from build123d import *

# Parameters (mm, degrees)
CROQUIS1_R              = 33
SALIENTE_EXTRUIR1_DEPTH = 10
VACIADO1_T              = -3
REDONDEO1_R             = 5
CORTAR_EXTRUIR1_REACH   = 49.728
CROQUIS2_R              = 1.25
CHAFL_N1_SIZE           = 1.6


with BuildPart() as part:
    # Croquis1 → Saliente-Extruir1 (new body)
    with BuildSketch(Plane.XY):
        Circle(CROQUIS1_R)
    extrude(amount=SALIENTE_EXTRUIR1_DEPTH)

    # Vaciado1
    vaciado1_openings = [part.faces().sort_by_distance(p)[0] for p in [
        (0, 0, 0),
    ]]
    offset(amount=VACIADO1_T, openings=vaciado1_openings, kind=Kind.INTERSECTION)

    # Redondeo1
    redondeo1_edges = [part.edges().sort_by_distance(p)[0] for p in [
        (-33, 0, 10),
        (-30, 0, 7),
    ]]
    fillet(redondeo1_edges, radius=REDONDEO1_R)

    # Croquis2 → Cortar-Extruir1 (cut, up to next)
    with BuildSketch(Plane.XY.offset(10), mode=Mode.PRIVATE) as cortar_extruir1_sk1:
        with Locations((14.041823927, -17.282568698)):
            Circle(CROQUIS2_R)
    cortar_extruir1_tool1 = extrude(cortar_extruir1_sk1.sketch, amount=-CORTAR_EXTRUIR1_REACH, mode=Mode.PRIVATE) & part.part
    # Croquis2 → Cortar-Extruir1 (cut, up to next)
    with BuildSketch(Plane.XY.offset(10), mode=Mode.PRIVATE) as cortar_extruir1_sk2:
        with Locations((19.215864901, 11.252134735)):
            Circle(CROQUIS2_R)
    cortar_extruir1_tool2 = extrude(cortar_extruir1_sk2.sketch, amount=-CORTAR_EXTRUIR1_REACH, mode=Mode.PRIVATE) & part.part
    # Croquis2 → Cortar-Extruir1 (cut, up to next)
    with BuildSketch(Plane.XY.offset(10), mode=Mode.PRIVATE) as cortar_extruir1_sk3:
        with Locations((-19.215864901, -11.252134735)):
            Circle(CROQUIS2_R)
    cortar_extruir1_tool3 = extrude(cortar_extruir1_sk3.sketch, amount=-CORTAR_EXTRUIR1_REACH, mode=Mode.PRIVATE) & part.part
    # Croquis2 → Cortar-Extruir1 (cut, up to next)
    with BuildSketch(Plane.XY.offset(10), mode=Mode.PRIVATE) as cortar_extruir1_sk4:
        with Locations((-14.041823927, 17.282568698)):
            Circle(CROQUIS2_R)
    cortar_extruir1_tool4 = extrude(cortar_extruir1_sk4.sketch, amount=-CORTAR_EXTRUIR1_REACH, mode=Mode.PRIVATE) & part.part
    add(cortar_extruir1_tool1.solids().sort_by_distance((14.041824, -17.282569, 10))[0], mode=Mode.SUBTRACT)
    add(cortar_extruir1_tool2.solids().sort_by_distance((19.215865, 11.252135, 10))[0], mode=Mode.SUBTRACT)
    add(cortar_extruir1_tool3.solids().sort_by_distance((-19.215865, -11.252135, 10))[0], mode=Mode.SUBTRACT)
    add(cortar_extruir1_tool4.solids().sort_by_distance((-14.041824, 17.282569, 10))[0], mode=Mode.SUBTRACT)

    # Chaflán1
    chafl_n1_edges = [part.edges().sort_by_distance(p)[0] for p in [
        (12.791823927, -17.282568698, 10),
        (17.965864901, 11.252134735, 10),
        (-20.465864901, -11.252134735, 10),
        (-15.291823927, 17.282568698, 10),
    ]]
    chamfer(chafl_n1_edges, length=CHAFL_N1_SIZE)


solid = part.part
Verification items for the finished model (mm, model axes). A direction names the side the tool comes from. Round coordinates to 2 decimals unless told otherwise and drop trailing zeros. Loops run counter-clockwise (first coordinate to the right, second up) from the corner with the lowest first, then second, coordinate; pieces in that order, holes last. Notation, with made-up numbers: (82, 56.25) - (132, 56.25) arc R21 ccw to (132, 66.25) - close; hole circle Ø6 at (14, -37). An arc over 180 degrees is marked (long way). Answer in a Markdown table with one row per item. Add a question column.
Q1. Section check C-C on z = 3. Enter the section's corners in (x, y), plus the area to 3 significant figures.
Q2. Tool access check on faces 5 (the face through (-29.97, 1.32, 0.99)), 6 (the face through (13.12, -16.44, 7.71)). Record the directions out of +Z, -Z, +X, -X, +Y, -Y that give a thin tool (end or side, any length) a straight path to the whole face; none if there is none.
Q3. Gauge pin test, flat ends, axial feed: pin 1 (5 mm diameter, centred on y = 23.5, z = 3, fed in from -X); pin 2 (25 mm diameter, centred on x = 0.5, y = 6.5, fed in from -Z); pin 3 (3 mm diameter, centred on x = -19.22, y = -11.25, fed in from +Z); pin 4 (1.5 mm diameter, centred on x = 14.04, y = -17.28, fed in from -Z). Record the tip position at first contact, or that the pin passes through.
Q4. Section check A-A on x = 0. Enter the section's corners in (y, z).
Q5. Release check for a two-part mould opening along Y. For faces 1 (the face through (20.37, 10.77, 7.71)), 2 (the face through (30.5, -12.6, 2.5)), 3 (the face through (0, 0, 7)), 4 (the face through (15, -27, 0)) record: pulls with the +Y half, pulls with the -Y half, needs draft (parallel to the pull), parting line crosses it, or undercut.
Q6. Material ranges on line 1 (Z direction, x = 0.5, y = 10.5); line 2 (Y direction, x = -15, z = 3); line 3 (Y direction, x = -27.5, z = 8), recorded low to high.
Found:
| question | item | result |
|---|---|---|
| 1 | outline | circle Ø66 at (0, 0); hole circle Ø59.8 at (0, 0) |
| 1 | area | 613 mm² |
| 2 | face 5 | -Z |
| 2 | face 6 | +Z, -Z |
| 3 | pin 1 | stops at x = -25.46 |
| 3 | pin 2 | stops at z = 7 |
| 3 | pin 3 | stops at z = 8.65 |
| 3 | pin 4 | passes through |
| 4 | outline | (-33, 0) - (-30, 0) - (-30, 2) arc R5 cw to (-25, 7) - (25, 7) arc R5 cw to (30, 2) - (30, 0) - (33, 0) - (33, 5) arc R5 ccw to (28, 10) - (-28, 10) arc R5 ccw to (-33, 5) - close |
| 5 | face 1 | undercut |
| 5 | face 2 | parting line crosses it |
| 5 | face 3 | undercut |
| 5 | face 4 | needs draft |
| 6 | line 1 | z = 7 to 10 |
| 6 | line 2 | y = -29.39 to -25.86, 25.86 to 29.39 |
| 6 | line 3 | y = -16.36 to 16.36 |
